```python
from build123d import *

# Parameters (mm, degrees)
SKETCH_1_W          = 11
SKETCH_1_H          = 40
EXTRUDE_1_DEPTH     = 13
SKETCH_2_W          = 40
SKETCH_2_H          = 1.5
EXTRUDE_2_DEPTH     = 48
SKETCH_3_W          = 12
SKETCH_3_H          = 0.5
EXTRUDE_3_DEPTH     = 0.7
SKETCH_4_W          = 20
SKETCH_4_H          = 0.495112862
EXTRUDE_4_DEPTH     = 0.7
CUT_EXTRUDE_1_DEPTH = 6
SKETCH_10_R         = 2.1
CUT_EXTRUDE_2_DEPTH = 9
CUT_EXTRUDE_3_DEPTH = 2
CUT_EXTRUDE_4_DEPTH = 2
SKETCH_17_W         = 1
SKETCH_17_H         = 20
EXTRUDE_6_DEPTH     = 2
SKETCH_21_W         = 6
SKETCH_21_H         = 13
EXTRUDE_8_DEPTH     = 13
SKETCH_23_R         = 2.1
CUT_EXTRUDE_7_DEPTH = 6
SKETCH_25_W         = 14
SKETCH_25_H         = 9.6
CUT_EXTRUDE_8_DEPTH = 11


with BuildPart() as part:
    # 草图1 → 凸台-拉伸1 (new body)
    with BuildSketch(Plane(origin=(0, 0, 0), x_dir=(1, 0, 0), z_dir=(0, 1, 0))):
        with Locations((-36.060761024, 1.454759243)):
            Rectangle(SKETCH_1_W, SKETCH_1_H)
        Polygon((17.439238976, -18.545240757), (-30.560761024, -18.545240757), (-41.560761024, -18.545240757), (-41.560761024, -20.545240757), (28.439238976, -20.545240757), (28.439238976, -18.545240757), align=None)
        with Locations((22.939238976, 1.454759243)):
            Rectangle(SKETCH_1_W, SKETCH_1_H)
    extrude(amount=EXTRUDE_1_DEPTH)

    # 草图2 → 凸台-拉伸2 (add)
    with BuildSketch(Plane(origin=(-30.560761024, 0, 0), x_dir=(0, 0, -1), z_dir=(1, 0, 0))):
        with Locations((1.454759243, 0.75)):
            Rectangle(SKETCH_2_W, SKETCH_2_H)
    extrude(amount=EXTRUDE_2_DEPTH)

    # 草图3 → 凸台-拉伸3 (add)
    with BuildSketch(Plane(origin=(-30.560761024, 0, 0), x_dir=(0, 0, -1), z_dir=(1, 0, 0))):
        with Locations((-5.453399323, 5.35)):
            Rectangle(SKETCH_3_W, SKETCH_3_H)
        with Locations((-5.453399323, 3.25)):
            Rectangle(SKETCH_3_W, SKETCH_3_H)
    extrude(amount=EXTRUDE_3_DEPTH)

    # 草图4 → 凸台-拉伸4 (add)
    with BuildSketch(Plane.ZY.offset(-17.439238976)):
        with Locations((8.545240757, 3.152443569)):
            Rectangle(SKETCH_4_W, SKETCH_4_H)
        with Locations((8.545240757, 5.247556431)):
            Rectangle(SKETCH_4_W, SKETCH_4_H)
    extrude(amount=EXTRUDE_4_DEPTH)

    # 草图5 → 切除-拉伸1 (cut)
    with BuildSketch(Plane(origin=(0, 0, 0), x_dir=(-1, 0, 0), z_dir=(0, -1, 0))):
        Polygon((-27.439238976, -12.097422285), (-27.439238976, -17.0626346), (-23.139238976, -19.545240757), (-18.839238976, -17.0626346), (-18.839238976, -12.097422285), (-23.139238976, -9.614816127), align=None)
        Polygon((31.960761024, -12.097422285), (31.960761024, -17.0626346), (36.260761024, -19.545240757), (40.560761024, -17.0626346), (40.560761024, -12.097422285), (36.260761024, -9.614816127), align=None)
        Polygon((31.960761024, 15.972153085), (31.960761024, 11.00694077), (36.260761024, 8.524334613), (40.560761024, 11.00694077), (40.560761024, 15.972153085), (36.260761024, 18.454759243), align=None)
    extrude(amount=-CUT_EXTRUDE_1_DEPTH, mode=Mode.SUBTRACT)

    # 草图10 → 切除-拉伸2 (cut)
    with BuildSketch(Plane.XZ.offset(-6)):
        with BuildLine():
            ThreePointArc((-34.160761024, -13.489546928), (-34.775836783, -12.004622687), (-36.260761024, -11.389546928))
            Line((-36.260761024, -11.389546928), (-36.260761024, -15.589546928))
            ThreePointArc((-36.260761024, -15.589546928), (-34.775836783, -14.974471168), (-34.160761024, -13.489546928))
        make_face()
        with BuildLine():
            Line((-36.260761024, -15.589546928), (-36.260761024, -11.389546928))
            ThreePointArc((-36.260761024, -11.389546928), (-38.360761024, -13.489546928), (-36.260761024, -15.589546928))
        make_face()
        with BuildLine():
            ThreePointArc((-34.160761024, 14.580028442), (-34.775836783, 16.064952683), (-36.260761024, 16.680028442))
            Line((-36.260761024, 16.680028442), (-36.260761024, 12.480028442))
            ThreePointArc((-36.260761024, 12.480028442), (-34.775836783, 13.095104202), (-34.160761024, 14.580028442))
        make_face()
        with BuildLine():
            Line((-36.260761024, 12.480028442), (-36.260761024, 16.680028442))
            ThreePointArc((-36.260761024, 16.680028442), (-38.360761024, 14.580028442), (-36.260761024, 12.480028442))
        make_face()
        with Locations(Location((23.139238976, 14.580028442, 0), (0, 0, 270))):
            Circle(SKETCH_10_R)
    extrude(amount=-CUT_EXTRUDE_2_DEPTH, mode=Mode.SUBTRACT)

    # 草图12 → 切除-拉伸3 (cut)
    with BuildSketch(Plane.XY.offset(20.545240757)):
        with BuildLine():
            Line((-27.310761024, 3.325), (-22.810761024, 3.325))
            ThreePointArc((-22.810761024, 3.325), (-19.310761024, 6.825), (-22.810761024, 10.325))
            Line((-22.810761024, 10.325), (-27.310761024, 10.325))
            ThreePointArc((-27.310761024, 10.325), (-30.810761024, 6.825), (-27.310761024, 3.325))
        make_face()
    extrude(amount=-CUT_EXTRUDE_3_DEPTH, mode=Mode.SUBTRACT)

    # 草图13 → 切除-拉伸4 (cut)
    with BuildSketch(Plane.XY.offset(20.545240757)):
        Polygon((-18.245761024, 13), (-18.210761024, 5.01), (-7.063003257, 5.01), (-7.065761024, 13), align=None)
    extrude(amount=-CUT_EXTRUDE_4_DEPTH, mode=Mode.SUBTRACT)

    # 草图17 → 凸台-拉伸6 (add)
    with BuildSketch(Plane(origin=(0, 13, 0), x_dir=(1, 0, 0), z_dir=(0, 1, 0))):
        with Locations((18.939238976, 11.439097948)):
            Rectangle(SKETCH_17_W, SKETCH_17_H)
    extrude(amount=EXTRUDE_6_DEPTH)

    # 草图21 → 凸台-拉伸8 (add)
    with BuildSketch(Plane(origin=(0, 0, -21.454759243), x_dir=(-1, 0, 0), z_dir=(0, 0, -1))):
        with Locations((38.560761024, 6.5)):
            Rectangle(SKETCH_21_W, SKETCH_21_H)
    extrude(amount=EXTRUDE_8_DEPTH)

    # 草图23 → 切除-拉伸7 (cut)
    with BuildSketch(Plane(origin=(-35.560761024, 0, 0), x_dir=(0, 0, -1), z_dir=(1, 0, 0))):
        with Locations((26.954759243, 7.5)):
            Circle(SKETCH_23_R)
    extrude(amount=-CUT_EXTRUDE_7_DEPTH, mode=Mode.SUBTRACT)

    # 草图25 → 切除-拉伸8 (cut)
    with BuildSketch(Plane(origin=(28.439238976, 0, 0), x_dir=(0, 0, -1), z_dir=(1, 0, 0))):
        with Locations((10.424759243, 8.2)):
            Rectangle(SKETCH_25_W, SKETCH_25_H)
    extrude(amount=-CUT_EXTRUDE_8_DEPTH, mode=Mode.SUBTRACT)


solid = part.part
```
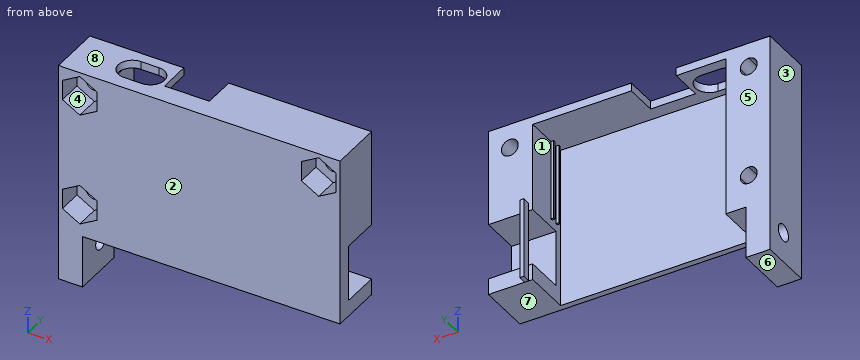
Check sheet for the modelled part. Datum: model origin and axes. Units: mm. Face numbers are marked on the shaded views. A direction names the side the tool comes from. Coordinates: 2 decimals unless noted, no trailing zeros. Order: outer loops, then holes, each group sorted by start corner. A loop starts at its lowest first (then second) coordinate and runs counter-clockwise, first axis right, second up. Notation, with made-up numbers: M -7.5,61 L 46.5,61 A22 cw 46.5,92 Z; hole C 37.25,54.25 d3. An arc over 180 degrees is marked long. Write each question's results on one line, items separated by ' | '. Start each with the question number.
1. Cross-section at A-A on z = -5. Record the cut outline in (x, y).
2. Cross-section at B-B on z = 5. Record the cut outline in (x, y), and give its area (3 significant figures).
3. Cross-section at D-D on z = -27. Record the cut outline in (x, y).
4. Access from +Z, -Z, +X, -X, +Y, -Y to the whole of each face (thin tool, end or side, straight path). Record for the marked faces 4, 5, 6, 7 and 8.
5. Material ranges on probe 1 along X at (y, z) = (7.75, -2); probe 2 along X at (y, z) = (9, 13); probe 3 along Z at (x, y) = (23.5, 12.25), recorded low to high.
6. Mould release check, pull along X, two halves, no side actions. Record for the marked faces 1, 2 and 3: +X half, -X half, draft (parallel to the pull), parting line (faces both ways), or undercut.
7. Go/stop test with flat-tipped pins: P1, Ø5.5, axis at y = 7.5, z = -26.95, coming from the -X side; P2, Ø6.5, axis at y = 3.5, z = -29.5, coming from the +X side; P3, Ø2, axis at x = -13, z = -10, coming from the +Y side; P4, Ø10, axis at x = -13, z = 14, coming from the +Y side. Record where each tip stops, or that it passes through.
8. Cross-section at C-C on x = 12. Record the cut outline in (y, z).
Checks:
1) outline: M -41.56,0 L 28.44,0 L 28.44,3.4 L 17.44,3.4 L 17.44,1.5 L -30.56,1.5 L -30.56,13 L -41.56,13 Z; M 18.44,13 L 19.44,13 L 19.44,15 L 18.44,15 Z
2) outline: M -41.56,0 L 28.44,0 L 28.44,13 L 17.44,13 L 17.44,5.5 L 16.74,5.5 L 16.74,5 L 17.44,5 L 17.44,3.4 L 16.74,3.4 L 16.74,2.9 L 17.44,2.9 L 17.44,1.5 L -30.56,1.5 L -30.56,3 L -29.86,3 L -29.86,3.5 L -30.56,3.5 L -30.56,5.1 L -29.86,5.1 L -29.86,5.6 L -30.56,5.6 L -30.56,13 L -41.56,13 Z | area: 359 mm²
3) outline: M -41.56,0 L -35.56,0 L -35.56,5.4 L -41.56,5.4 Z; M -41.56,9.6 L -35.56,9.6 L -35.56,13 L -41.56,13 Z
4) face 4: -Y | face 5: +Z, -Z, -X, +Y | face 6: -Z, +X, -X, +Y, -Y | face 7: -Z, +X, +Y, -Y | face 8: +Z, +X, -X, +Y, -Y
5) probe 1: x = -41.56 to -30.56, 17.44 to 28.44 | probe 2: x = -41.56 to -37.64, -34.88 to -30.56, 17.44 to 21.76, 24.52 to 28.44 | probe 3: z = -21.45 to -17.42, -3.42 to 12.51, 16.65 to 20.55
6) face 1: undercut | face 2: draft | face 3: -X half
7) P1: stops at x = -41.56 | P2: stops at x = -35.56 | P3: stops at y = 1.5 | P4: stops at y = 5.01
8) outline: M 0,-21.45 L 1.5,-21.45 L 1.5,18.55 L 13,18.55 L 13,20.55 L 0,20.55 Z
